from build123d import *

# Parameters (mm, degrees)
F0_R     = 36.930663
F1_DEPTH = 77.47
F2_W     = 95.02399
F2_H     = 75.079672
F3_DEPTH = 25.4


with BuildPart() as f1:
    # F0 (on Front) → F1 (new body)
    with BuildSketch(Plane.XZ):
        with Locations((4.31927, 0)):
            Circle(F0_R)
    extrude(amount=F1_DEPTH)

    # F2 (on Front) → F3 (join)
    with BuildSketch(Plane.XZ):
        with Locations((-16.125284, -0.623651)):
            Rectangle(F2_W, F2_H)
    extrude(amount=-F3_DEPTH)


solid = f1.part
Geometry: final body of the model. Coordinates: model frame, mm. A direction names the side the tool comes from. Give positions to 0.01 mm unless a question says otherwise; leave off trailing zeros. Write each loop counter-clockwise with the first axis right and the second up, starting at its lowest first coordinate (ties: lowest second). Pieces come first, ordered by that corner, then holes. Notation, with made-up numbers: (18, -6.75) -> (73, -6.75) arc R12 ccw to (73, 1.25) -> close; hole circle Ø3 at (59, -18.5). An arc over 180 degrees is marked (long way). Answer as a JSON object with one key per item and string values.
1. Access query for faces 4 (the flat face through (31.387, 13, -1)), 5 (the flat face through (25, 0, 33)), 6 (the flat face through (-17, 13, 36.916)), 7 (the flat face through (-17, 13, -38.163)), 8 (the cylindrical face through (-3.69, -38.19, -36.05)). Directions: +Z, -Z, +X, -X, +Y, -Y. A direction counts if a zero-diameter tool reaches every point of the face in a straight line with its end or side. Return the directions, or none.
Ans:
{"face 4": "+Z, -Z, +X, +Y", "face 5": "+Z, +X, -Y", "face 6": "+Z, +X, -X, +Y, -Y", "face 7": "-Z, +X, -X, +Y, -Y", "face 8": "-Y"}
2. Cut plane A-A on z = 0. Output: boundary loops of the cut face in (x, y), and give its area (3 significant figures).
Ans:
{"outline": "(-63.64, 0) -> (-32.61, 0) -> (-32.61, -77.47) -> (41.25, -77.47) -> (41.25, 0) -> (31.39, 0) -> (31.39, 25.4) -> (-63.64, 25.4) -> close", "area": "8,140 mm^2"}
3. Contact query for flat-ended pins moving along their axis: pin 1 (6 mm diameter, centred on y = -43, z = -19.5, fed in from -X); pin 2 (2 mm diameter, centred on x = -35.5, y = -21, fed in from -Z); pin 3 (20.5 mm diameter, centred on x = -30, y = 16.5, fed in from +Z); pin 4 (1 mm diameter, centred on y = -13.5, z = -8.5, fed in from +X). Output: stop coordinate, or through.
Ans:
{"pin 1": "stops at x = -28.72", "pin 2": "passes through", "pin 3": "stops at z = 36.92", "pin 4": "stops at x = 40.37"}
4. Cut plane D-D on z = -23.5. Output: boundary loops of the cut face in (x, y), and give its area (3 significant figures).
Ans:
{"outline": "(-63.64, 0) -> (-24.17, 0) -> (-24.17, -77.47) -> (32.81, -77.47) -> (32.81, 0) -> (31.39, 0) -> (31.39, 25.4) -> (-63.64, 25.4) -> close", "area": "6,830 mm^2"}
5. Cut plane B-B on x = -50.5. Output: boundary loops of the cut face in (y, z).
Ans:
{"outline": "(0, -38.16) -> (25.4, -38.16) -> (25.4, 36.92) -> (0, 36.92) -> close"}
6. Ray query, probe 1 along Y at (x, z) = (-40.5, -22); probe 2 along Y at (x, z) = (32, -0.5); probe 3 along Z at (x, y) = (4, -56.5). Return the intervals inside material, ascending. Write a range as from..to.
Ans:
{"probe 1": "y = 0..25.4", "probe 2": "y = -77.47..0", "probe 3": "z = -36.93..36.93"}
7. Mould query, pull axis Y, two halves, no side actions, for faces 1 (the flat face through (-17, 25.4, 0)), 2 (the flat face through (4, -77.47, 1)), 3 (the flat face through (-63.637, 13, -1)). Classes: pulls with the +Y half, pulls with the -Y half, needs draft (parallel to the pull), parting line crosses it, or undercut.
Ans:
{"face 1": "pulls with the +Y half", "face 2": "pulls with the -Y half", "face 3": "needs draft"}
8. Cut plane C-C on y = -14.5. Output: boundary loops of the cut face in (x, z), and give its area (3 significant figures).
Ans:
{"outline": "circle Ø73.86 at (4.32, 0)", "area": "4,280 mm^2"}
